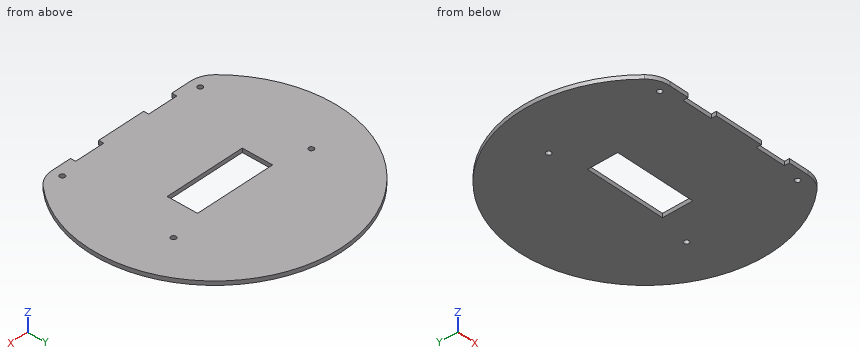
from build123d import *

# Parameters (mm, degrees)
SKETCH1_R           = 125
BOSS_EXTRUDE1_DEPTH = 4
CUT_EXTRUDE2_START  = -10
CUT_EXTRUDE2_DEPTH  = 10
FILLET1_R           = 25
SKETCH6_W           = 30
SKETCH6_H           = 5
CUT_EXTRUDE5_DEPTH  = 5
SKETCH7_R           = 2.5
CUT_EXTRUDE6_DEPTH  = 177.821944339
SKETCH8_W           = 80
SKETCH8_H           = 30
CUT_EXTRUDE7_DEPTH  = 177.821944339


with BuildPart() as part:
    # Sketch1 → Boss-Extrude1 (new body)
    with BuildSketch(Plane.XY):
        Circle(SKETCH1_R)
    extrude(amount=BOSS_EXTRUDE1_DEPTH)

    # Sketch3 → Cut-Extrude2 (cut)
    with BuildSketch(Plane.XY.offset(4).offset(CUT_EXTRUDE2_START)):
        with BuildLine():
            Line((-83.915537646, -92.645466924), (83.915537646, -92.645466924))
            ThreePointArc((83.915537646, -92.645466924), (0, -125), (-83.915537646, -92.645466924))
        make_face()
    extrude(amount=CUT_EXTRUDE2_DEPTH, mode=Mode.SUBTRACT)

    # Fillet1
    fillet1_edges = [part.edges().sort_by_distance(p)[0] for p in [
        (83.915537646, -92.645466924, 2),
        (-83.915537646, -92.645466924, 2),
    ]]
    fillet(fillet1_edges, radius=FILLET1_R)

    # Sketch6 → Cut-Extrude5 (cut)
    with BuildSketch(Plane.XY.offset(4)):
        with Locations((39, -90.145466924)):
            Rectangle(SKETCH6_W, SKETCH6_H)
        with Locations((-39, -90.145466924)):
            Rectangle(SKETCH6_W, SKETCH6_H)
    extrude(amount=-CUT_EXTRUDE5_DEPTH, mode=Mode.SUBTRACT)

    # Sketch7 → Cut-Extrude6 (cut, through all)
    with BuildSketch(Plane.XY.offset(4)):
        with Locations((73.5, -82.645466924)):
            Circle(SKETCH7_R)
        with Locations((73.5, 27.354533076)):
            Circle(SKETCH7_R)
        with Locations((-73.5, 27.354533076)):
            Circle(SKETCH7_R)
        with Locations((-73.5, -82.645466924)):
            Circle(SKETCH7_R)
    extrude(amount=-CUT_EXTRUDE6_DEPTH, mode=Mode.SUBTRACT)

    # Sketch8 → Cut-Extrude7 (cut, through all)
    with BuildSketch(Plane.XY.offset(4)):
        with Locations((0, 5.074477417)):
            Rectangle(SKETCH8_W, SKETCH8_H)
    extrude(amount=-CUT_EXTRUDE7_DEPTH, mode=Mode.SUBTRACT)


solid = part.part
Work out the finished part from the listing and answer in its coordinate system (mm). Give positions to 0.01 mm unless a question says otherwise; leave off trailing zeros. Loops run counter-clockwise (first coordinate to the right, second up) from the corner with the lowest first, then second, coordinate; pieces in that order, holes last. Notation, with made-up numbers: (58, 34) -> (110, 34) arc R10 ccw to (110, 47) -> close; hole circle Ø1 at (36, 16). An arc over 180 degrees is marked (long way). Use a Markdown table: item, result. Add a question column.
1. Section A-A on x = 0 is taken. Determine the outline of the cut face in (y, z).
2. Flat-ended cylindrical pins translate along their axes: pin 1 Ø1.2 at (x, z) = (-11.5, 2.5) entering from +Y; pin 2 Ø4.5 at (x, y) = (73.5, -82.65) entering from +Z; pin 3 Ø2 at (y, z) = (-91, 1.5) entering from -X; pin 4 Ø2 at (y, z) = (-67.5, 2.5) entering from +X. Find the tip coordinate at first contact, or state that the pin passes through.
3. Find the intervals of material crossed by probe 1 along Y at (x, z) = (3, 2.9); probe 2 along Y at (x, z) = (-73.5, 1.15); probe 3 along Y at (x, z) = (14, 2.4), in increasing order.
4. Section B-B on y = 0 is taken. Determine the outline of the cut face in (x, z), and give its area (3 significant figures).
5. Section C-C on z = 1.7 is taken. Determine the outline of the cut face in (x, y), and give its area (3 significant figures).
6. Section D-D on y = -35 is taken. Determine the outline of the cut face in (x, z).
Results below:
| question | item | result |
|---|---|---|
| 1 | outline | (-92.65, 0) -> (-9.93, 0) -> (-9.93, 4) -> (-92.65, 4) -> close; (20.07, 0) -> (125, 0) -> (125, 4) -> (20.07, 4) -> close |
| 2 | pin 1 | stops at y = 124.52 |
| 2 | pin 2 | passes through |
| 2 | pin 3 | stops at x = -84.84 |
| 2 | pin 4 | stops at x = 105.84 |
| 3 | probe 1 | y = -92.65 to -9.93, 20.07 to 124.96 |
| 3 | probe 2 | y = -92.65 to -85.15, -80.15 to 24.85, 29.85 to 101.11 |
| 3 | probe 3 | y = -92.65 to -9.93, 20.07 to 124.21 |
| 4 | outline | (-125, 0) -> (-40, 0) -> (-40, 4) -> (-125, 4) -> close; (40, 0) -> (125, 0) -> (125, 4) -> (40, 4) -> close |
| 4 | area | 680 mm^2 |
| 5 | outline | (-92.06, -84.56) arc R25 ccw to (-73.65, -92.65) -> (-54, -92.65) -> (-54, -87.65) -> (-24, -87.65) -> (-24, -92.65) -> (24, -92.65) -> (24, -87.65) -> (54, -87.65) -> (54, -92.65) -> (73.65, -92.65) arc R25 ccw to (92.06, -84.56) arc R125 ccw (long way) to start; hole circle Ø5 at (-73.5, -82.65); hole circle Ø5 at (-73.5, 27.35); hole (-40, -9.93) -> (40, -9.93) -> (40, 20.07) -> (-40, 20.07) -> close; hole circle Ø5 at (73.5, -82.65); hole circle Ø5 at (73.5, 27.35) |
| 5 | area | 42,600 mm^2 |
| 6 | outline | (-120, 0) -> (120, 0) -> (120, 4) -> (-120, 4) -> close |
